Autodesk Inventor part; units mm, degrees
ref_plane "Work Plane1" through (74.6218, 1.0791, 0) normal (1, 0, 0) x (0, 0, -1)
ref_plane "Work Plane2" through (-19.3782, 27.0791, 0) normal (0, -1, 0) x (1, 0, 0)
ref_plane "YZ Plane" through (0, 0, 0) normal (1, 0, 0) x (0, 1, 0)
sketch "Sketch1" plane through (0, 0, 0) normal (0, 0, 1) x (1, 0, 0)
  line L0 (-19.3782, 63.0791) -> (164.6218, 63.0791)
  line L1 (174.6218, 53.0791) -> (174.6218, 1.0791)
  line L2 (164.6218, -8.9209) -> (-19.3782, -8.9209)
  line L3 (-29.3782, 1.0791) -> (-29.3782, 53.0791)
  arc A0 (-19.3782, 63.0791) -> (-29.3782, 53.0791) centre (-19.3782, 53.0791) ccw
  arc A1 (-29.3782, 1.0791) -> (-19.3782, -8.9209) centre (-19.3782, 1.0791) ccw
  arc A2 (164.6218, -8.9209) -> (174.6218, 1.0791) centre (164.6218, 1.0791) ccw
  arc A3 (174.6218, 53.0791) -> (164.6218, 63.0791) centre (164.6218, 53.0791) ccw
  point P0 (0, 0)
  point P1 (-29.3782, 63.0791)
  point P2 (174.6218, -8.9209)
  point P3 (-29.3782, -8.9209)
  dimension "d0" = 204
  dimension "d1" = 72
  dimension "d2" = 10
extrude "Extrusion1" add sketch "Sketch1" along normal blind 6
sketch "Sketch4" plane through (0, 0, 6) normal (0, 0, 1) x (1, 0, 0)
  circle A0 centre (-4.3782, 5.0791) radius 2
  circle A1 centre (-19.3782, 14.5791) radius 2
  circle A2 centre (-4.3782, 49.0791) radius 2
  circle A3 centre (-19.3782, 39.5791) radius 2
  line L0 (164.6218, 63.0791) -> (-19.3782, 63.0791)
  line L1 (72.6218, 63.0791) -> (72.6218, -8.9209)
  line L2 (-19.3782, -8.9209) -> (164.6218, -8.9209)
  circle A4 centre (151.6218, 5.0791) radius 2
  circle A5 centre (151.6218, 49.0791) radius 2
  line L3 (-29.3782, 53.0791) -> (-29.3782, 1.0791)
  point P0 (0, 0)
  dimension "d17" = 4
  dimension "d19" = 4
  dimension "d38" = 14
  dimension "d39" = 14
  dimension "d40" = 25
  dimension "d41" = 25
  dimension "d43" = 156
  dimension "d44" = 156
  dimension "d45" = 79
extrude "Extrusion4" cut sketch "Sketch4" against normal blind 6 contours A0 | A2 | A4 | A5
ref_plane "Work Plane1" through (74.6218, 1.0791, 0) normal (1, 0, 0) x (0, 0, -1)
ref_plane "Work Plane2" through (-19.3782, 27.0791, 0) normal (0, -1, 0) x (1, 0, 0)
sketch "Sketch5" plane through (0, 0, 0) normal (0, 0, -1) x (-1, 0, 0)
  line L0 (-41.6218, -8.9209) -> (-72.6218, -8.9209)
  line L1 (-72.6218, -8.9209) -> (-72.6218, 21.0791)
  line L2 (-72.6218, 21.0791) -> (-41.6218, 21.0791)
  line L3 (-41.6218, 21.0791) -> (-41.6218, -8.9209)
  line L4 (19.3782, -8.9209) -> (-164.6218, -8.9209)
  line L5 (-164.6218, 63.0791) -> (19.3782, 63.0791)
  line L6 (-72.6218, -8.9209) -> (-103.6218, -8.9209)
  line L7 (-103.6218, -8.9209) -> (-103.6218, 21.0791)
  line L8 (-103.6218, 21.0791) -> (-72.6218, 21.0791)
  line L9 (-72.6218, 21.0791) -> (-72.6218, -8.9209)
  line L10 (-43.8163, 63.0791) -> (-72.6218, 63.0791)
  line L11 (-72.6218, 63.0791) -> (-72.6218, 33.0791)
  line L12 (-72.6218, 33.0791) -> (-53.8163, 33.0791)
  line L13 (-43.8163, 32.0791) -> (-43.8163, 63.0791)
  line L14 (-72.6218, 33.0791) -> (-93.6218, 33.0791)
  line L15 (-103.6218, 31.0791) -> (-103.6218, 63.0791)
  line L16 (-103.6218, 63.0791) -> (-72.6218, 63.0791)
  line L17 (-72.6218, 63.0791) -> (-72.6218, 33.0791)
  line L18 (-41.6218, -8.9209) -> (-6.6218, -8.9209)
  line L19 (-43.8163, 63.0791) -> (-11.7113, 63.0791)
  line L20 (-103.6218, -8.9209) -> (-138.6218, -8.9209)
  line L21 (-103.6218, 63.0791) -> (-138.6218, 63.0791)
  line L22 (-43.8163, 63.0791) -> (-28.8163, 63.0791)
  line L23 (-28.8163, 63.0791) -> (-28.8163, 51.444)
  line L24 (-43.8163, 32.0791) -> (-43.8163, 63.0791)
  line L25 (-103.6218, 63.0791) -> (-118.6218, 63.0791)
  line L26 (-118.6218, 63.0791) -> (-118.6218, 50.444)
  line L27 (-103.6218, 31.0791) -> (-103.6218, 63.0791)
  line L28 (-72.6218, -8.9209) -> (-72.6218, 21.0791)
  line L29 (-72.6218, 33.0791) -> (-72.6218, 63.0791)
  line L30 (-28.8163, 51.444) -> (-28.8163, 43.0791)
  line L31 (-38.8163, 33.0791) -> (-53.8163, 33.0791)
  line L32 (-93.6218, 33.0791) -> (-108.6218, 33.0791)
  line L33 (-118.6218, 43.0791) -> (-118.6218, 50.444)
  arc A0 (-38.8163, 33.0791) -> (-28.8163, 43.0791) centre (-38.8163, 43.0791) ccw
  arc A1 (-118.6218, 43.0791) -> (-108.6218, 33.0791) centre (-108.6218, 43.0791) ccw
  line L34 (29.3782, 1.0791) -> (29.3782, 53.0791)
  point P0 (0, 0)
  dimension "d25" = 31
  dimension "d26" = 30
  dimension "d27" = 31
  dimension "d28" = 30
  dimension "d29" = 35
  dimension "d30" = 35
  dimension "d46" = 15
  dimension "d47" = 15
  dimension "d48" = 10
  dimension "d61" = 102
extrude "Extrusion5" cut sketch "Sketch5" against normal blind 6 contours L5 L15 L32 A1 L33 L26 | L5 L11 L14 L32 L15 | L5 L13 L31 L12 L11 | L5 L23 L30 A0 L31 L13
ref_plane "Work Plane3" through (-19.3782, 27.0791, 6) normal (0, 1, 0) x (1, 0, 0)
mirror "Mirror1" about plane through (-19.3782, 27.0791, 6) normal (0, 1, 0) of "Extrusion5"
fillet "Fillet1" radius 10 4 edges at (118.6218, 63.0791, 3) (28.8163, 63.0791, 3) (28.8163, -8.9209, 3) (118.6218, -8.9209, 3)
sketch "Sketch7" plane through (0, 0, 0) normal (0, 0, -1) x (-1, 0, 0)
  circle A0 centre (13.8782, -1.9209) radius 2
  circle A1 centre (13.8782, 56.0791) radius 2
  circle A2 centre (-161.1218, 56.0791) radius 2
  circle A3 centre (-161.1218, -1.9209) radius 2
  line L0 (-28.8163, 53.0791) -> (-28.8163, 43.0791)
  line L1 (-28.8163, 11.0791) -> (-28.8163, 1.0791)
  line L2 (-118.6218, 1.0791) -> (-118.6218, 11.0791)
  line L3 (-118.6218, 43.0791) -> (-118.6218, 53.0791)
  point P0 (0, 0)
  point P1 (-161.1218, 5.0791)
  dimension "d49" = 4
  dimension "d50" = 4
  dimension "d54" = 7
  dimension "d57" = 42.6945
  dimension "d58" = 42.6945
  dimension "d59" = 42.5
  dimension "d60" = 42.5
extrude "Extrusion6" cut sketch "Sketch7" against normal blind 6
sketch "Sketch8" plane through (0, 0, 6) normal (0, 0, 1) x (1, 0, 0)
  line L0 (-29.3782, 1.0791) -> (-29.3782, 53.0791)
  line L1 (-29.3782, 27.0791) -> (174.6218, 27.0791)
  line L2 (174.6218, 53.0791) -> (174.6218, 1.0791)
  circle A0 centre (45.6218, 27.0791) radius 2
  circle A1 centre (99.6218, 27.0791) radius 2
  point P0 (0, 0)
  dimension "d62" = 4
  dimension "d63" = 4
  dimension "d64" = 75
  dimension "d65" = 75
extrude "Extrusion7" cut sketch "Sketch8" against normal blind 6
properties part number "top plate" material "UHMW, White"
Geometry: final body of the model. Coordinates: model frame, mm. A direction names the side the tool comes from. Round coordinates to 2 decimals unless told otherwise and drop trailing zeros. Loops run counter-clockwise (first coordinate to the right, second up) from the corner with the lowest first, then second, coordinate; pieces in that order, holes last. Notation, with made-up numbers: (49.25, -13.75) -> (72.25, -13.75) arc R21 cw to (72.25, 7.25) -> close; hole circle Ø4 at (-5, -0.5). An arc over 180 degrees is marked (long way). Use one line per item in the form item = value.
Item 1: Cut plane D-D on x = 111. Output: boundary loops of the cut face in (y, z).
Evaluation:
outline = (20.79, 0) -> (33.37, 0) -> (33.37, 6) -> (20.79, 6) -> close
Item 2: Cut plane C-C on x = 80.5. Output: boundary loops of the cut face in (y, z), then the cut area to 3 significant figures.
Evaluation:
outline = (21.08, 0) -> (33.08, 0) -> (33.08, 6) -> (21.08, 6) -> close
area = 72.0 mm2
Item 3: Access query for faces 1 (the flat face through (147, -8.921, 3)), 2 (the cylindrical face through (121.6, 60.2, 3)), 3 (the flat face through (28.816, 6, 3)). Directions: +Z, -Z, +X, -X, +Y, -Y. A direction counts if a zero-diameter tool reaches every point of the face in a straight line with its end or side. Return the directions, or none.
Evaluation:
face_1 = +Z, -Z, +X, -X, -Y
face_2 = +Z, -Z, +Y
face_3 = +Z, -Z, -Y
Item 4: Material intervals for probe 1 along X at (y, z) = (11.5, 1.75); probe 2 along Y at (x, z) = (43, 1.3); probe 3 along X at (y, z) = (15.5, 4.2), sorted ascending.
Evaluation:
probe_1 = -29.38 to 28.83, 118.61 to 174.62
probe_2 = 21.08 to 33.08
probe_3 = -29.38 to 29.85, 117.59 to 174.62
Item 5: Cut plane A-A on y = 36. Output: boundary loops of the cut face in (x, z).
Evaluation:
outline = (-29.38, 0) -> (31.75, 0) -> (31.75, 6) -> (-29.38, 6) -> close; (115.68, 0) -> (174.62, 0) -> (174.62, 6) -> (115.68, 6) -> close
Item 6: Contact query for flat-ended pins moving along their axis: pin 1 Ø1.5 at (x, z) = (107.5, 2) entering from +Y; pin 2 Ø3 at (x, y) = (151.62, 49.08) entering from -Z; pin 3 Ø6.5 at (x, y) = (99.62, 27.08) entering from +Z; pin 4 Ø2 at (x, z) = (65.5, 4) entering from -Y. Output: stop coordinate, or through.
Evaluation:
pin_1 = 33.08
pin_2 = through
pin_3 = 6
pin_4 = 21.08
Item 7: Cut plane B-B on z = 1.5. Give the number of separate pieces and of enclosed holes in the cut face, then the cut area to 3 significant figures.
Evaluation:
separate_pieces = 1
enclosed_holes = 10
area = 9,090 mm2
Item 8: Draft query along X for faces 4 (the flat face through (146, 63.079, 3)), 5 (the cylindrical face through (-3.455, 47.305, 3.042)), 6 (the cylindrical face through (171.61, 60.23, 2.96)). Return one class per face: released by +X, released by -X, zero draft, split by the parting line, or undercut.
Evaluation:
face_4 = zero draft
face_5 = undercut
face_6 = released by +X
